Read the model definition and answer for the solid it produces. Units are mm, in the model's axes. A direction names the side the tool comes from. Coordinates: 2 decimals unless noted, no trailing zeros. Write each loop counter-clockwise with the first axis right and the second up, starting at its lowest first coordinate (ties: lowest second). Pieces come first, ordered by that corner, then holes. Notation, with made-up numbers: (47.25, 79) -> (80.25, 79) arc R21 ccw to (80.25, 92) -> close; hole circle Ø6 at (6.25, -31). An arc over 180 degrees is marked (long way). Return JSON: item names as keys, results as strings.
from build123d import *

# Parameters (mm, degrees)
SKETCH1_W           = 38
SKETCH1_H           = 73.8
BOSS_EXTRUDE1_DEPTH = 1.5
SKETCH2_W           = 38
SKETCH2_H           = 73.8
SKETCH2_W_2         = 34
SKETCH2_H_2         = 69.8
BOSS_EXTRUDE2_DEPTH = 3.8
FILLET1_R           = 1
SKETCH3_R           = 1
CUT_EXTRUDE1_DEPTH  = 2.5
SKETCH4_W           = 7.6
SKETCH4_H           = 1.82
CUT_EXTRUDE2_DEPTH  = 2.5
SKETCH5_W           = 9.5
SKETCH5_H           = 2
CUT_EXTRUDE3_DEPTH  = 2.5
LPATTERN1_COUNT     = 2
LPATTERN1_PITCH     = 56
SKETCH6_W           = 34
SKETCH6_H           = 61.8
SKETCH6_W_2         = 9.5
SKETCH6_H_2         = 2
BOSS_EXTRUDE3_DEPTH = 3.4
SKETCH7_W           = 32
SKETCH7_H           = 59.8
CUT_EXTRUDE5_DEPTH  = 3.4
SKETCH9_W           = 15
SKETCH9_H           = 0.9
CUT_EXTRUDE7_DEPTH  = 37
SKETCH10_W          = 10
SKETCH10_H          = 0.5
CUT_EXTRUDE8_DEPTH  = 7


with BuildPart() as part:
    # Sketch1 → Boss-Extrude1 (new body)
    with BuildSketch(Plane(origin=(0, 0, 0), x_dir=(1, 0, 0), z_dir=(0, 1, 0))):
        Rectangle(SKETCH1_W, SKETCH1_H)
    extrude(amount=BOSS_EXTRUDE1_DEPTH)

    # Sketch2 → Boss-Extrude2 (add)
    with BuildSketch(Plane(origin=(0, 1.5, 0), x_dir=(1, 0, 0), z_dir=(0, 1, 0))):
        Rectangle(SKETCH2_W, SKETCH2_H)
        Rectangle(SKETCH2_W_2, SKETCH2_H_2, mode=Mode.SUBTRACT)
    extrude(amount=BOSS_EXTRUDE2_DEPTH)

    # Fillet1
    fillet1_edges = [part.edges().sort_by_distance(p)[0] for p in [
        (19, 2.65, 36.9),
        (-19, 2.65, 36.9),
        (-19, 2.65, -36.9),
        (19, 2.65, -36.9),
    ]]
    fillet(fillet1_edges, radius=FILLET1_R)

    # Sketch3 → Cut-Extrude1 (cut, through all)
    with BuildSketch(Plane(origin=(0, 1.5, 0), x_dir=(1, 0, 0), z_dir=(0, 1, 0))):
        with Locations((-16, 33.9)):
            Circle(SKETCH3_R)
        with Locations((16, 33.9)):
            Circle(SKETCH3_R)
    cut_extrude1 = extrude(amount=-CUT_EXTRUDE1_DEPTH, mode=Mode.SUBTRACT)

    # Mirror1: Cut-Extrude1 across plane
    add(cut_extrude1.mirror(Plane.XY), mode=Mode.SUBTRACT)

    # Sketch4 → Cut-Extrude2 (cut, through all)
    with BuildSketch(Plane(origin=(0, 1.5, 0), x_dir=(1, 0, 0), z_dir=(0, 1, 0))):
        with Locations((-3.8, 33.99)):
            Rectangle(SKETCH4_W, SKETCH4_H)
    extrude(amount=-CUT_EXTRUDE2_DEPTH, mode=Mode.SUBTRACT)

    # Sketch5 → Cut-Extrude3 (cut, through all)
    with BuildSketch(Plane(origin=(0, 1.5, 0), x_dir=(1, 0, 0), z_dir=(0, 1, 0))):
        with Locations((-10.3, 28.1)):
            Rectangle(SKETCH5_W, SKETCH5_H)
        with Locations((0, 28.1)):
            Rectangle(SKETCH5_W, SKETCH5_H)
        with Locations((10.3, 28.1)):
            Rectangle(SKETCH5_W, SKETCH5_H)
    cut_extrude3 = extrude(amount=-CUT_EXTRUDE3_DEPTH, mode=Mode.SUBTRACT)

    # LPattern1: Cut-Extrude3 ×2
    with Locations(*[(0, 0, i * LPATTERN1_PITCH) for i in range(1, LPATTERN1_COUNT)]):
        add(cut_extrude3, mode=Mode.SUBTRACT)

    # Sketch6 → Boss-Extrude3 (add)
    with BuildSketch(Plane.XZ):
        Rectangle(SKETCH6_W, SKETCH6_H)
        with Locations((-10.3, 27.9)):
            Rectangle(SKETCH6_W_2, SKETCH6_H_2, mode=Mode.SUBTRACT)
        with Locations((0, 27.9)):
            Rectangle(SKETCH6_W_2, SKETCH6_H_2, mode=Mode.SUBTRACT)
        with Locations((10.3, 27.9)):
            Rectangle(SKETCH6_W_2, SKETCH6_H_2, mode=Mode.SUBTRACT)
        with Locations((-10.3, -28.1)):
            Rectangle(SKETCH6_W_2, SKETCH6_H_2, mode=Mode.SUBTRACT)
        with Locations((0, -28.1)):
            Rectangle(SKETCH6_W_2, SKETCH6_H_2, mode=Mode.SUBTRACT)
        with Locations((10.3, -28.1)):
            Rectangle(SKETCH6_W_2, SKETCH6_H_2, mode=Mode.SUBTRACT)
    extrude(amount=BOSS_EXTRUDE3_DEPTH)

    # Sketch7 → Cut-Extrude5 (cut)
    with BuildSketch(Plane(origin=(0, 1.5, 0), x_dir=(1, 0, 0), z_dir=(0, 1, 0))):
        Rectangle(SKETCH7_W, SKETCH7_H)
    extrude(amount=-CUT_EXTRUDE5_DEPTH, mode=Mode.SUBTRACT)

    # Sketch9 → Cut-Extrude7 (cut, through all)
    with BuildSketch(Plane(origin=(17, 0, 0), x_dir=(0, 0, -1), z_dir=(1, 0, 0))):
        with Locations((23.4, -2.95)):
            Rectangle(SKETCH9_W, SKETCH9_H)
    extrude(amount=-CUT_EXTRUDE7_DEPTH, mode=Mode.SUBTRACT)

    # Sketch10 → Cut-Extrude8 (cut)
    with BuildSketch(Plane.ZY.offset(17)):
        with Locations((-4.1, -3.15)):
            Rectangle(SKETCH10_W, SKETCH10_H)
    extrude(amount=-CUT_EXTRUDE8_DEPTH, mode=Mode.SUBTRACT)


solid = part.part
1. Consider L1, parallel to X at y = 0.6, z = 33.9; L2, parallel to Z at x = -2, y = -1.5; L3, parallel to X at y = 0.95, z = -33.9. Determine where each line is inside the solid, lowest interval first.
Taken from the geometry:
{"L1": "x = -19 to -17, -15 to 15, 17 to 19", "L2": "z = -30.9 to -29.9, 29.9 to 30.9", "L3": "x = -19 to -17, -15 to -7.6, 0 to 15, 17 to 19"}
2. Flat-ended cylindrical pins translate along their axes: pin 1 Ø1.6 at (y, z) = (-2.5, 28) entering from -X; pin 2 Ø12 at (x, z) = (-6.5, 17) entering from +Y; pin 3 Ø1.2 at (x, y) = (-0.5, -2.5) entering from -Z. Find the tip coordinate at first contact, or state that the pin passes through.
Taken from the geometry:
{"pin 1": "stops at x = -17", "pin 2": "stops at y = -1.9", "pin 3": "stops at z = -30.9"}
3. The part is cut by section A-A (x = 2.5). Determine the outline of the cut face in (y, z).
Taken from the geometry:
{"outline": "(-3.4, -15.9) -> (-2.5, -15.9) -> (-2.5, -27.1) -> (-1.9, -27.1) -> (-1.9, 26.9) -> (-3.4, 26.9) -> close; (-3.4, 28.9) -> (-1.9, 28.9) -> (-1.9, 29.9) -> (1.5, 29.9) -> (1.5, 34.9) -> (5.3, 34.9) -> (5.3, 36.9) -> (0, 36.9) -> (0, 30.9) -> (-3.4, 30.9) -> close; (-2.5, -30.9) -> (0, -30.9) -> (0, -36.9) -> (5.3, -36.9) -> (5.3, -34.9) -> (1.5, -34.9) -> (1.5, -29.9) -> (-1.9, -29.9) -> (-1.9, -29.1) -> (-2.5, -29.1) -> close"}
4. The part is cut by section B-B (z = 18.5). Determine the outline of the cut face in (x, y).
Taken from the geometry:
{"outline": "(-19, 0) -> (-17, 0) -> (-17, -3.4) -> (17, -3.4) -> (17, 0) -> (19, 0) -> (19, 5.3) -> (17, 5.3) -> (17, 1.5) -> (16, 1.5) -> (16, -1.9) -> (-16, -1.9) -> (-16, 1.5) -> (-17, 1.5) -> (-17, 5.3) -> (-19, 5.3) -> close"}
5. For a pull along Z with two mould halves and no side action, classify faces 4 (the face through (0, 0, -29.9)), 5 (the face through (0, -1, -30.9)), 6 (the face through (15.05, -3, 28)) as +Z half, -Z half, draft (parallel to the pull), parting line (faces both ways), or undercut.
Taken from the geometry:
{"face 4": "undercut", "face 5": "-Z half", "face 6": "undercut"}
6. The part is cut by section D-D (z = -24.5). Determine the outline of the cut face in (x, y).
Taken from the geometry:
{"outline": "(-19, 0) -> (-17, 0) -> (-17, -2.5) -> (17, -2.5) -> (17, 0) -> (19, 0) -> (19, 5.3) -> (17, 5.3) -> (17, 1.5) -> (16, 1.5) -> (16, -1.9) -> (-16, -1.9) -> (-16, 1.5) -> (-17, 1.5) -> (-17, 5.3) -> (-19, 5.3) -> close"}
7. The part is cut by section C-C (x = -13.5). Count the separate pieces of the cut face and the enclosed holes in it, then the cut area to 3 significant figures.
Taken from the geometry:
{"separate pieces": "3", "enclosed holes": "0", "area": "110 mm2"}
8. A tool of negligible diameter and unlimited length cuts with its end or side. For faces 1 (the face through (10, -3, 28.9)), 2 (the face through (0, 3, -34.9)), 3 (the face through (-14, -2.9, -4)), from which of +Z, -Z, +X, -X, +Y, -Y can it reach the whole face along a straight path? Write none if from no direction.
Taken from the geometry:
{"face 1": "+Y, -Y", "face 2": "+Y", "face 3": "-X, -Y"}
